Part model, mm, in its own coordinate system. A direction names the side the tool comes from. Give positions to 0.01 mm unless a question says otherwise; leave off trailing zeros. Write each loop counter-clockwise with the first axis right and the second up, starting at its lowest first coordinate (ties: lowest second). Pieces come first, ordered by that corner, then holes. Notation, with made-up numbers: M -20.5,-30 L 36.5,-30 A20 cw 36.5,-16 Z; hole C 84,86.5 d1. An arc over 180 degrees is marked long. Answer as CSV lines item,"result". Start each with the question number.
1) Slice it at A-A, the plane y = 450. Give the cut face in (x, z), plus the area to 3 significant figures.
2) Mould opens along X. For faces 3 (the cylindrical face through (-393.05, 450.84, 50.97)), 4 (the flat face through (-396.5, 237, -20)), 5 (the flat face through (-5, 473, -22)), 6 (the flat face through (-5, 237, -213)) say: pulls with the +X half, pulls with the -X half, needs draft (parallel to the pull), parting line crosses it, or undercut.
3) Tool access for faces 1 (the flat face through (-389.5, 237, -16)), 2 (the flat face through (396.5, 237, -20)): list every direction of +Z, -Z, +X, -X, +Y, -Y with a clear straight run to the whole face (end or side of a thin tool).
4) Slice it at B-B, the plane z = 70. Give the cut face in (x, y).
5) Slice it at D-D, the plane x = -188. Give the cut face in (y, z).
6) Pin check, flat tips, straight feed: pin 1 Ø8 at (x, y) = (158.5, 128.5) entering from +Z; pin 2 Ø5 at (x, z) = (-366.5, 90) entering from -Y. Stop position of each tip, or through.
7) Wall check: line 1 along X through (y, z) = (4, -120) (3 decimals); line 2 along Y through (x, z) = (71, -88.5); line 3 along X through (y, z) = (239.5, 154.5). Give the ranges that are in metal, low to high. Write a range as from..to.
8) Slice it at C-C, the plane z = -81.5. Give the cut face in (x, y).
```python
from build123d import *

# Parameters (mm, degrees)
CROQUIS1_W              = 793
CROQUIS1_H              = 440
SALIENTE_EXTRUIR1_DEPTH = 480
VACIADO1_T              = -7
CROQUIS2_R              = 12.7
CORTAR_EXTRUIR1_DEPTH   = 80
CROQUIS3_R              = 6.35
CORTAR_EXTRUIR2_DEPTH   = 10
CROQUIS5_R              = 6.35
CORTAR_EXTRUIR4_DEPTH   = 10
CROQUIS6_R              = 19.05
CORTAR_EXTRUIR5_DEPTH   = 848
CROQUIS8_R              = 12.7
CORTAR_EXTRUIR6_DEPTH   = 10
CROQUIS9_W              = 35.052267511
CROQUIS9_H              = 245.374735938
SALIENTE_EXTRUIR2_DEPTH = 7
CROQUIS15_R             = 3.175
CORTAR_EXTRUIR10_DEPTH  = 10
CROQUIS18_R             = 3.175
CROQUIS18_R_2           = 5.554937391
CORTAR_EXTRUIR12_DEPTH  = 10
CROQUIS19_W             = 793
CROQUIS19_H             = 480
CORTAR_EXTRUIR13_DEPTH  = 45
CROQUIS20_W             = 40.222844752
CROQUIS20_H             = 335.190372933
SALIENTE_EXTRUIR3_DEPTH = 7
CROQUIS22_W             = 754.715939893
CROQUIS22_H             = 447.32434432
SALIENTE_EXTRUIR4_DEPTH = 7


with BuildPart() as part:
    # Croquis1 → Saliente-Extruir1 (new body)
    with BuildSketch(Plane(origin=(0, 0, 0), x_dir=(1, 0, 0), z_dir=(0, 1, 0))):
        Rectangle(CROQUIS1_W, CROQUIS1_H)
    extrude(amount=SALIENTE_EXTRUIR1_DEPTH)

    # Vaciado1
    vaciado1_openings = [part.faces().sort_by_distance(p)[0] for p in [
        (0, 240, 220),
    ]]
    offset(amount=VACIADO1_T, openings=vaciado1_openings, kind=Kind.INTERSECTION)

    # Croquis2 → Cortar-Extruir1 (cut)
    with BuildSketch(Plane.XZ):
        with Locations(Location((-340.681431581, 41.288678468, 0), (0, 0, 270))):
            Circle(CROQUIS2_R)
    cortar_extruir1 = extrude(amount=-CORTAR_EXTRUIR1_DEPTH, mode=Mode.SUBTRACT)

    # Croquis3 → Cortar-Extruir2 (cut)
    with BuildSketch(Plane.XZ):
        with Locations(Location((-340.681431581, 81.288678468, 0), (0, 0, 270))):
            Circle(CROQUIS3_R)
    cortar_extruir2 = extrude(amount=-CORTAR_EXTRUIR2_DEPTH, mode=Mode.SUBTRACT)

    # Croquis5 → Cortar-Extruir4 (cut)
    with BuildSketch(Plane.XZ):
        with Locations(Location((-340.681431581, 121.288678468, 0), (0, 0, 270))):
            Circle(CROQUIS5_R)
    cortar_extruir4 = extrude(amount=-CORTAR_EXTRUIR4_DEPTH, mode=Mode.SUBTRACT)

    # Croquis6 → Cortar-Extruir5 (cut)
    with BuildSketch(Plane.ZY.offset(396.5)):
        with Locations((-130, 450)):
            Circle(CROQUIS6_R)
        with Locations((70, 450)):
            Circle(CROQUIS6_R)
    extrude(amount=-CORTAR_EXTRUIR5_DEPTH, mode=Mode.SUBTRACT)

    # Simetría1: Cortar-Extruir1, Cortar-Extruir2, Cortar-Extruir4 across plane
    add(cortar_extruir1.mirror(Plane(origin=(0, 0, 0), x_dir=(0, 0, 1), z_dir=(1, 0, 0))), mode=Mode.SUBTRACT)
    add(cortar_extruir2.mirror(Plane(origin=(0, 0, 0), x_dir=(0, 0, 1), z_dir=(1, 0, 0))), mode=Mode.SUBTRACT)
    add(cortar_extruir4.mirror(Plane(origin=(0, 0, 0), x_dir=(0, 0, 1), z_dir=(1, 0, 0))), mode=Mode.SUBTRACT)

    # Croquis8 → Cortar-Extruir6 (cut)
    with BuildSketch(Plane.XZ):
        with Locations(Location((340.681431581, -121.411321532, 0), (0, 0, 270))):
            Circle(CROQUIS8_R)
    extrude(amount=-CORTAR_EXTRUIR6_DEPTH, mode=Mode.SUBTRACT)

    # Croquis9 → Saliente-Extruir2 (add)
    with BuildSketch(Plane(origin=(0, 7, 0), x_dir=(1, 0, 0), z_dir=(0, 1, 0))):
        with Locations((-340.681431581, -81.288678468)):
            Rectangle(CROQUIS9_W, CROQUIS9_H)
    extrude(amount=-SALIENTE_EXTRUIR2_DEPTH)

    # Croquis15 → Cortar-Extruir10 (cut)
    with BuildSketch(Plane.XZ):
        with Locations(Location((-366.5, -120, 0), (0, 0, 270))):
            Circle(CROQUIS15_R)
        with Locations(Location((-366.5, 90, 0), (0, 0, 90))):
            Circle(CROQUIS15_R)
        with Locations(Location((366.5, -120, 0), (0, 0, 90))):
            Circle(CROQUIS15_R)
        with Locations(Location((366.5, 90, 0), (0, 0, 270))):
            Circle(CROQUIS15_R)
    extrude(amount=-CORTAR_EXTRUIR10_DEPTH, mode=Mode.SUBTRACT)

    # Croquis18 → Cortar-Extruir12 (cut)
    with BuildSketch(Plane.XY.offset(-213)):
        with Locations((-348, 438)):
            Circle(CROQUIS18_R)
        with Locations((0, 438)):
            Circle(CROQUIS18_R)
        with Locations((348, 438)):
            Circle(CROQUIS18_R)
        with Locations((348, 240)):
            Circle(CROQUIS18_R)
        with Locations((348, 42)):
            Circle(CROQUIS18_R)
        with Locations((0, 42)):
            Circle(CROQUIS18_R)
        with Locations((-348, 42)):
            Circle(CROQUIS18_R)
        with Locations((-348, 240)):
            Circle(CROQUIS18_R_2)
    extrude(amount=-CORTAR_EXTRUIR12_DEPTH, mode=Mode.SUBTRACT)

    # Croquis19 → Cortar-Extruir13 (cut)
    with BuildSketch(Plane.XY.offset(220)):
        with Locations((0, 240)):
            Rectangle(CROQUIS19_W, CROQUIS19_H)
    extrude(amount=-CORTAR_EXTRUIR13_DEPTH, mode=Mode.SUBTRACT)

    # Croquis20 → Saliente-Extruir3 (add)
    with BuildSketch(Plane.XZ):
        with Locations((336.531134424, -29.98561058)):
            Rectangle(CROQUIS20_W, CROQUIS20_H)
    extrude(amount=-SALIENTE_EXTRUIR3_DEPTH)

    # Croquis22 → Saliente-Extruir4 (add)
    with BuildSketch(Plane(origin=(0, 0, -220), x_dir=(-1, 0, 0), z_dir=(0, 0, -1))):
        with Locations((2.077532213, 243.10690677)):
            Rectangle(CROQUIS22_W, CROQUIS22_H)
    extrude(amount=-SALIENTE_EXTRUIR4_DEPTH)


solid = part.part
```
Found:
1,outline,"M -396.5,-220 L 396.5,-220 L 396.5,-149.05 L 389.5,-149.05 L 389.5,-213 L -389.5,-213 L -389.5,-149.05 L -396.5,-149.05 Z; M -396.5,-110.95 L -389.5,-110.95 L -389.5,50.95 L -396.5,50.95 Z; M -396.5,89.05 L -389.5,89.05 L -389.5,175 L -396.5,175 Z; M 389.5,-110.95 L 396.5,-110.95 L 396.5,50.95 L 389.5,50.95 Z; M 389.5,89.05 L 396.5,89.05 L 396.5,175 L 389.5,175 Z"
1,area,"9,920 mm²"
2,face 3,"needs draft"
2,face 4,"pulls with the -X half"
2,face 5,"undercut"
2,face 6,"undercut"
3,face 1,"+Z"
3,face 2,"+Z, -Z, +X, +Y, -Y"
4,outline,"M -396.5,0 L 396.5,0 L 396.5,430.95 L 389.5,430.95 L 389.5,7 L -389.5,7 L -389.5,430.95 L -396.5,430.95 Z; M -396.5,469.05 L -389.5,469.05 L -389.5,473 L 389.5,473 L 389.5,469.05 L 396.5,469.05 L 396.5,480 L -396.5,480 Z"
5,outline,"M 0,-220 L 480,-220 L 480,175 L 473,175 L 473,-213 L 7,-213 L 7,175 L 0,175 Z"
6,pin 1,"z = -213"
6,pin 2,"y = 473"
7,line 1,"-396.5..-369.675, -363.325..363.325, 369.675..396.5"
7,line 2,"0..7, 473..480"
7,line 3,"-396.5..-389.5, 389.5..396.5"
8,outline,"M -396.5,0 L 396.5,0 L 396.5,480 L -396.5,480 Z; hole M -389.5,7 L 389.5,7 L 389.5,473 L -389.5,473 Z"
